from build123d import *

# Parameters (mm, degrees)
SKETCH2_R = 50


with BuildPart() as part:
    # Sweep1: sweep along a path in Sketch1
    with BuildLine(Plane(origin=(0, 0, 0), x_dir=(0, 0, -1), z_dir=(1, 0, 0))) as sweep1_path:
        Line((-45, 0), (45, 0))
        Line((45, 0), (45, 85))
    # Sketch2 → Sweep1 (sweep)
    with BuildSketch(Plane.XY.offset(45)):
        Circle(SKETCH2_R)
    sweep1 = sweep(path=sweep1_path.line, transition=Transition.RIGHT)

    # Mirror2: Sweep1 across plane
    add(sweep1.mirror(Plane.XY.offset(-45)))


solid = part.part
CAD build for the part. Positions are in the model's coordinates, mm. A direction names the side the tool comes from. Coordinates: 2 decimals unless noted, no trailing zeros. Loops run counter-clockwise (first coordinate to the right, second up) from the corner with the lowest first, then second, coordinate; pieces in that order, holes last. Notation, with made-up numbers: (60, -29) - (89, -29) arc R24 cw to (89, 2) - close; hole circle Ø9 at (-9.5, -20). An arc over 180 degrees is marked (long way). Use one line per item in the form item = value. Start each with the question number.
1) Tool access for faces 1 (the face through (-1, 1, 45)), 2 (the face through (-49.95, 52.54, -47.2)): list every direction of +Z, -Z, +X, -X, +Y, -Y with a clear straight run to the whole face (end or side of a thin tool).
2) Band-saw the part on C-C (z = -106). Give the cut face in (x, y), and give its area (3 significant figures).
3) Flat gauge pins, fed straight in: pin 1 (6 mm diameter, centred on x = 38.5, z = -90.5, fed in from +Y); pin 2 (12 mm diameter, centred on x = -36, z = -102.5, fed in from -Y); pin 3 (8 mm diameter, centred on y = 6.5, z = -13.5, fed in from +X). Where does each tip first touch, or does it go through?
4) Band-saw the part on A-A (x = 0). Give the cut face in (y, z).
5) Band-saw the part on D-D (y = 75.5). Give the cut face in (x, z), and give its area (3 significant figures).
6) Drill centre lines: L1, parallel to Z at x = -1, y = 62; L2, parallel to X at y = 66, z = -44.5; L3, parallel to Y at x = 0.5, z = -66. Where is each one in solid material? Low to high. Write a range as from..to.
7) Band-saw the part on B-B (y = 38). Give the cut face in (x, z).
Check values:
q1.face_1 = +Z, +X, -X, +Y, -Y
q1.face_2 = +Y
q2.outline = circle Ø100 at (0, 0)
q2.area = 7,850 mm2
q3.pin_1 = 35.21
q3.pin_2 = -40
q3.pin_3 = 49.94
q4.outline = (-50, -135) - (50, -135) - (50, -95) - (85, -95) - (85, 5) - (50, 5) - (50, 45) - (-50, 45) - close
q5.outline = circle Ø100 at (0, -45)
q5.area = 7,850 mm2
q6.L1 = -94.99..4.99
q6.L2 = -50..50
q6.L3 = -50..85
q7.outline = (-32.5, -135) - (32.5, -135) - (32.5, -83) arc R50 ccw to (32.5, -7) - (32.5, 45) - (-32.5, 45) - (-32.5, -7) arc R50 ccw to (-32.5, -83) - close
